```python
from build123d import *

# Parameters (mm, degrees)
EXTRUDE_1_DEPTH     = 76
SKETCH_2_R          = 1.5
CUT_EXTRUDE_1_DEPTH = 76
SKETCH_3_R          = 2.5
CUT_EXTRUDE_2_DEPTH = 76


with BuildPart() as part:
    # 草图1 → 凸台-拉伸1 (new body)
    with BuildSketch(Plane(origin=(0, 0, 0), x_dir=(1, 0, 0), z_dir=(0, 1, 0))):
        Polygon((0, 0), (14, 0), (14, 14), (12, 14), (12, 2), (0, 2), align=None)
    extrude(amount=EXTRUDE_1_DEPTH)

    # 草图2 → 切除-拉伸1 (cut)
    with BuildSketch(Plane.XY):
        with Locations((4.2, 4.25)):
            Circle(SKETCH_2_R)
        with Locations((4.2, 71.75)):
            Circle(SKETCH_2_R)
    extrude(amount=-CUT_EXTRUDE_1_DEPTH, mode=Mode.SUBTRACT)

    # 草图3 → 切除-拉伸2 (cut)
    with BuildSketch(Plane(origin=(14, 0, 0), x_dir=(0, 0, -1), z_dir=(1, 0, 0))):
        with Locations((7, 23)):
            Circle(SKETCH_3_R)
        with Locations((7, 53)):
            Circle(SKETCH_3_R)
    extrude(amount=-CUT_EXTRUDE_2_DEPTH, mode=Mode.SUBTRACT)


solid = part.part
```
Could you check a few things on this model? Use its own coordinates, in mm. A direction names the side the tool comes from. Round coordinates to 2 decimals unless told otherwise and drop trailing zeros. Order: outer loops, then holes, each group sorted by start corner. A loop starts at its lowest first (then second) coordinate and runs counter-clockwise, first axis right, second up. Notation, with made-up numbers: (50, -21.5) -> (67, -21.5) arc R16 cw to (67, -5.5) -> close; hole circle Ø11 at (16, -24.75). An arc over 180 degrees is marked (long way). One line per question, with ' | ' between items.
Q1. If we section it at A-A on y = 71.75: Write out the boundary of the cut face in (x, z).
Computed values:
outline: (0, -2) -> (2.7, -2) -> (2.7, 0) -> (0, 0) -> close; (5.7, -2) -> (12, -2) -> (12, -14) -> (14, -14) -> (14, 0) -> (5.7, 0) -> close
Q2. Which directions (+Z, -Z, +X, -X, +Y, -Y) give clear straight access to the entire face, cutting with the end or side of a thin tool? Please do faces 1 (the face through (12, 37, -8)), 2 (the face through (5.006, 73.015, -0.986)).
Computed values:
face 1: -Z, -X, +Y, -Y | face 2: +Z, -Z
Q3. We'd pull the mould along Y, two halves only. Please class faces 3 (the face through (12.2, 0, -4.4)), 4 (the face through (13.014, 53.751, -9.385)), 5 (the face through (6, 37, -2)), 6 (the face through (13.01, 25.11, -8.34)): released by +Y, released by -Y, zero draft, split by the parting line, or undercut.
Computed values:
face 3: released by -Y | face 4: undercut | face 5: zero draft | face 6: undercut
Q4. If we section it at B-B on z = -7: Write out the boundary of the cut face in (x, y), plus the area to 3 significant figures.
Computed values:
outline: (12, 0) -> (14, 0) -> (14, 20.5) -> (12, 20.5) -> close; (12, 25.5) -> (14, 25.5) -> (14, 50.5) -> (12, 50.5) -> close; (12, 55.5) -> (14, 55.5) -> (14, 76) -> (12, 76) -> close | area: 132 mm²
Q5. If we section it at D-D on y = 23: Write out the boundary of the cut face in (x, z).
Computed values:
outline: (0, -2) -> (12, -2) -> (12, -4.5) -> (14, -4.5) -> (14, 0) -> (0, 0) -> close; (12, -14) -> (14, -14) -> (14, -9.5) -> (12, -9.5) -> close
Q6. If I drill on line 1 (Y direction, x = 4.2, z = -0.95); line 2 (Y direction, x = 13, z = -7); line 3 (X direction, y = 71.75, z = -1.6), over which ranges is the centre line in solid material (lowest first)? Write a range as from..to.
Computed values:
line 1: 0..2.75, 5.75..70.25, 73.25..76 | line 2: 0..20.5, 25.5..50.5, 55.5..76 | line 3: 0..2.7, 5.7..14
Q7. If we section it at C-C on x = 4.25: Write out the boundary of the cut face in (y, z).
Computed values:
outline: (0, -2) -> (2.75, -2) -> (2.75, 0) -> (0, 0) -> close; (5.75, -2) -> (70.25, -2) -> (70.25, 0) -> (5.75, 0) -> close; (73.25, -2) -> (76, -2) -> (76, 0) -> (73.25, 0) -> close
Q8. I'm going to push flat-ended pins straight in: pin 1 (4 mm diameter, centred on y = 60, z = -5.5, fed in from -X); pin 2 (3 mm diameter, centred on x = 10, y = 35.5, fed in from -Z); pin 3 (8 mm diameter, centred on x = 10.5, z = -4, fed in from -Y); pin 4 (2.5 mm diameter, centred on x = 4.2, y = 71.75, fed in from +Z). Where does each tip first touch, or does it pass through?
Computed values:
pin 1: x = 12 | pin 2: z = -2 | pin 3: y = 0 | pin 4: through
